CAD build for the part. Positions are in the model's coordinates, mm. Coordinates: 2 decimals unless noted, no trailing zeros. Loops run counter-clockwise (first coordinate to the right, second up) from the corner with the lowest first, then second, coordinate; pieces in that order, holes last. Notation, with made-up numbers: (45, 17.5) -> (76, 17.5) arc R5 ccw to (76, 24.5) -> close; hole circle Ø8 at (55, -12.5). An arc over 180 degrees is marked (long way). Write each question's results on one line, items separated by ' | '.
```python
from build123d import *

# Parameters (mm, degrees)
EXTRUDE_1_DEPTH     = 5
SKETCH_3_W          = 40
SKETCH_3_H          = 25
EXTRUDE_2_DEPTH     = 5
SKETCH_2_R          = 2
SKETCH_2_R_2        = 1
SKETCH_2_R_3        = 1.5
SKETCH_2_R_4        = 7.5
SKETCH_2_W          = 2
SKETCH_2_H          = 40
SKETCH_2_W_2        = 11.8
SKETCH_2_H_2        = 22.5
CUT_EXTRUDE_1_DEPTH = 10
FILLET_2_R          = 5


with BuildPart() as part:
    # 草图1 → 凸台-拉伸1 (new body)
    with BuildSketch(Plane(origin=(0, 0, 0), x_dir=(1, 0, 0), z_dir=(0, 1, 0))):
        Polygon((0, 0), (150, 0), (150, 100), (150, 200), (0, 200), (0, 100), align=None)
    extrude(amount=EXTRUDE_1_DEPTH)

    # 草图3 → 凸台-拉伸2 (add)
    with BuildSketch(Plane(origin=(0, 5, 0), x_dir=(1, 0, 0), z_dir=(0, 1, 0))):
        with Locations((75, -12.5)):
            Rectangle(SKETCH_3_W, SKETCH_3_H)
    extrude(amount=-EXTRUDE_2_DEPTH)

    # 草图2 → 切除-拉伸1 (cut)
    with BuildSketch(Plane(origin=(0, 5, 0), x_dir=(1, 0, 0), z_dir=(0, 1, 0))):
        with Locations(Location((11, 38, 0), (0, 0, 270))):
            Circle(SKETCH_2_R)
        with Locations(Location((25, 38, 0), (0, 0, 270))):
            Circle(SKETCH_2_R)
        with Locations(Location((11, 22, 0), (0, 0, 270))):
            Circle(SKETCH_2_R)
        with Locations(Location((25, 22, 0), (0, 0, 270))):
            Circle(SKETCH_2_R)
        with Locations(Location((125, 22, 0), (0, 0, 90))):
            Circle(SKETCH_2_R)
        with Locations(Location((139, 22, 0), (0, 0, 90))):
            Circle(SKETCH_2_R)
        with Locations(Location((139, 38, 0), (0, 0, 90))):
            Circle(SKETCH_2_R)
        with Locations(Location((125, 38, 0), (0, 0, 90))):
            Circle(SKETCH_2_R)
        with Locations(Location((75, -17.35, 0), (0, 0, 270))):
            Circle(SKETCH_2_R_2)
        with Locations(Location((75, 9.85, 0), (0, 0, 270))):
            Circle(SKETCH_2_R_2)
        with Locations(Location((49.5, 70, 0), (0, 0, 270))):
            Circle(SKETCH_2_R_3)
        with Locations(Location((49.5, 121, 0), (0, 0, 90))):
            Circle(SKETCH_2_R_3)
        with Locations(Location((100.5, 121, 0), (0, 0, 270))):
            Circle(SKETCH_2_R_3)
        with Locations(Location((100.5, 70, 0), (0, 0, 90))):
            Circle(SKETCH_2_R_3)
        with Locations(Location((110, 165, 0), (0, 0, 270))):
            Circle(SKETCH_2_R_3)
        with Locations(Location((147, 165, 0), (0, 0, 270))):
            Circle(SKETCH_2_R_3)
        with Locations(Location((110, 104, 0), (0, 0, 270))):
            Circle(SKETCH_2_R_3)
        with Locations(Location((147, 104, 0), (0, 0, 270))):
            Circle(SKETCH_2_R_3)
        with Locations(Location((5, 115.5, 0), (0, 0, 270))):
            Circle(SKETCH_2_R_3)
        with Locations(Location((42, 115.5, 0), (0, 0, 270))):
            Circle(SKETCH_2_R_3)
        with Locations(Location((42, 78.5, 0), (0, 0, 270))):
            Circle(SKETCH_2_R_3)
        with Locations(Location((5, 78.5, 0), (0, 0, 270))):
            Circle(SKETCH_2_R_3)
        with Locations(Location((6, 194, 0), (0, 0, 270))):
            Circle(SKETCH_2_R_3)
        with Locations(Location((84.6, 194, 0), (0, 0, 270))):
            Circle(SKETCH_2_R_3)
        with Locations(Location((84.6, 142, 0), (0, 0, 270))):
            Circle(SKETCH_2_R_3)
        with Locations(Location((6, 142, 0), (0, 0, 270))):
            Circle(SKETCH_2_R_3)
        with Locations(Location((45, 131, 0), (0, 0, 270))):
            Circle(SKETCH_2_R_3)
        with Locations(Location((105, 131, 0), (0, 0, 90))):
            Circle(SKETCH_2_R_3)
        with Locations(Location((33, 5, 0), (0, 0, 270))):
            Circle(SKETCH_2_R_3)
        with Locations(Location((33, 47, 0), (0, 0, 270))):
            Circle(SKETCH_2_R_3)
        with Locations(Location((117, 47, 0), (0, 0, 270))):
            Circle(SKETCH_2_R_3)
        with Locations(Location((117, 5, 0), (0, 0, 270))):
            Circle(SKETCH_2_R_3)
        with Locations(Location((105, 161, 0), (0, 0, 270))):
            Circle(SKETCH_2_R_3)
        with Locations(Location((45, 161, 0), (0, 0, 270))):
            Circle(SKETCH_2_R_3)
        with Locations(Location((15, 70, 0), (0, 0, 270))):
            Circle(SKETCH_2_R_4)
        with Locations(Location((15, 130, 0), (0, 0, 270))):
            Circle(SKETCH_2_R_4)
        with Locations((101, 95.5)):
            Rectangle(SKETCH_2_W, SKETCH_2_H)
        with Locations((75, -3.75)):
            Rectangle(SKETCH_2_W_2, SKETCH_2_H_2)
        with Locations((49, 95.5)):
            Rectangle(SKETCH_2_W, SKETCH_2_H)
    extrude(amount=-CUT_EXTRUDE_1_DEPTH, mode=Mode.SUBTRACT)

    # 圆角2
    fillet_2_edges = [part.edges().sort_by_distance(p)[0] for p in [
        (0, 2.5, -200),
        (150, 2.5, -200),
        (150, 2.5, 0),
        (0, 2.5, 0),
        (55, 2.5, 0),
        (95, 2.5, 0),
        (95, 2.5, 25),
        (55, 2.5, 25),
    ]]
    fillet(fillet_2_edges, radius=FILLET_2_R)


solid = part.part
```
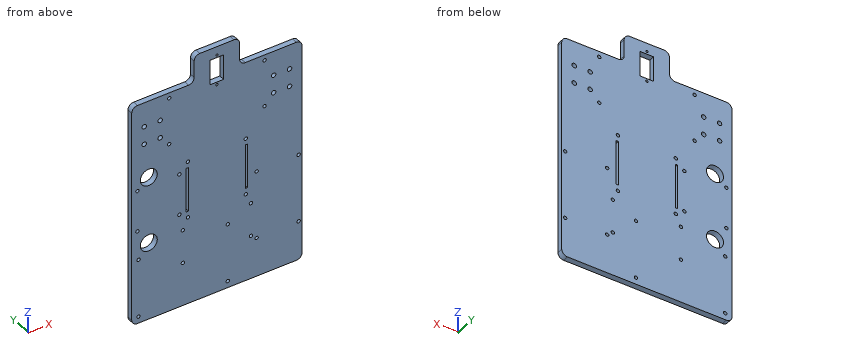
Q1. Drop flat-ended pins along their axis: pin 1 (1.5 mm diameter, centred on x = 23.5, y = 2, fed in from +Z); pin 2 (1.5 mm diameter, centred on y = 2.5, z = 0, fed in from +X); pin 3 (3 mm diameter, centred on x = 93.5, y = 4, fed in from +Z). Give the stop position or say it passes through.
Results are:
pin 1: z = 0 | pin 2: x = 147.63 | pin 3: z = 24.58
Q2. Cut at A-A on z = 7.5. Write the cut outline in (x, y).
Results are:
outline: (55, 0) -> (69.1, 0) -> (69.1, 5) -> (55, 5) -> close; (80.9, 0) -> (95, 0) -> (95, 5) -> (80.9, 5) -> close
Q3. Cut at D-D on x = 131.5. Write the cut outline in (y, z), and give its area (3 significant figures).
Results are:
outline: (0, -200) -> (5, -200) -> (5, 0) -> (0, 0) -> close | area: 1,000 mm^2
Q4. Cut at B-B on z = -90.5. Write the cut outline in (x, y).
Results are:
outline: (0, 0) -> (48, 0) -> (48, 5) -> (0, 5) -> close; (50, 0) -> (100, 0) -> (100, 5) -> (50, 5) -> close; (102, 0) -> (150, 0) -> (150, 5) -> (102, 5) -> close
Q5. Wall check: L1, parallel to X at y = 1.9, z = -22; L2, parallel to X at y = 3.1, z = -70; L3, parallel to X at y = 2.15, z = -121. Give the ranges that are in metal, low to high. Write a range as from..to.
Results are:
L1: 0..9, 13..23, 27..123, 127..137, 141..150 | L2: 0..7.5, 22.5..48, 51..99, 102..150 | L3: 0..48, 51..99, 102..150
Q6. Cut at C-C on y = 1.9. Give the number of separate pieces and of enclosed holes in the cut face, and give its area (3 significant figures).
Results are:
separate pieces: 1 | enclosed holes: 39 | area: 29,900 mm^2
